```python
from build123d import *

# Parameters (mm, degrees)
SKETCH002_R  = 2.25
PAD002_DEPTH = 2
SKETCH003_W  = 7
SKETCH003_H  = 2
PAD003_DEPTH = 2
SKETCH004_W  = 32
SKETCH004_H  = 12
POCKET_DEPTH = 2


with BuildPart() as part:
    # Sketch002 → Pad002 (new body)
    with BuildSketch(Plane.XY):
        with BuildLine():
            Line((22.5, 12.5), (22.5, -12.5))
            Line((22.5, -12.5), (-5.5, -12.5))
            Line((-5.5, -12.5), (-5.5, -16.5))
            ThreePointArc((-15.5, -16.5), (-10.5, -21.5), (-5.5, -16.5))
            Line((-15.5, -12.5), (-15.5, -16.5))
            Line((-22.5, -12.5), (-15.5, -12.5))
            Line((-22.5, 12.5), (-22.5, -12.5))
            Line((-15.5, 12.5), (-22.5, 12.5))
            Line((-15.5, 16.5), (-15.5, 12.5))
            ThreePointArc((-5.5, 16.5), (-10.5, 21.5), (-15.5, 16.5))
            Line((-5.5, 16.5), (-5.5, 12.5))
            Line((-5.5, 12.5), (22.5, 12.5))
        make_face()
        with Locations((-10.5, 16.5)):
            Circle(SKETCH002_R, mode=Mode.SUBTRACT)
        with Locations((-10.5, -16.5)):
            Circle(SKETCH002_R, mode=Mode.SUBTRACT)
    extrude(amount=PAD002_DEPTH)

    # Sketch003 (on Face16 of Pad002) → Pad003 (join)
    with BuildSketch(Plane.XY.offset(2)):
        with Locations((19, -11.5)):
            Rectangle(SKETCH003_W, SKETCH003_H)
        Polygon((20.5, 10.5), (15.5, 10.5), (15.5, 12.5), (22.5, 12.5), (22.5, -0.5), (20.5, -0.5), align=None)
        Polygon((-15.5, 12.5), (-22.5, 12.5), (-22.5, -12.5), (-15.5, -12.5), (-15.5, -10.5), (-20.5, -10.5), (-20.5, 10.5), (-15.5, 10.5), align=None)
    extrude(amount=PAD003_DEPTH)

    # Sketch004 (on Face4 of Pad003) → Pocket (cut)
    with BuildSketch(Plane.XY.offset(2)):
        Rectangle(SKETCH004_W, SKETCH004_H)
    extrude(amount=-POCKET_DEPTH, mode=Mode.SUBTRACT)


solid = part.part
```
Verification items for the finished model (mm, model axes). A direction names the side the tool comes from. Coordinates: 2 decimals unless noted, no trailing zeros. Loops run counter-clockwise (first coordinate to the right, second up) from the corner with the lowest first, then second, coordinate; pieces in that order, holes last. Notation, with made-up numbers: (20, -36.75) -> (65, -36.75) arc R22 cw to (65, -20.75) -> close; hole circle Ø6 at (81.25, -39). An arc over 180 degrees is marked (long way). Put each result on its own line as item: value.
1. Gauge pin test, flat ends, axial feed: P1, Ø2, axis at y = 14, z = 1, coming from the -X side; P2, Ø4, axis at x = 15, y = -7, coming from the +Z side; P3, Ø2, axis at x = -20.5, z = 1, coming from the -Y side. Record the tip position at first contact, or that the pin passes through.
Result set:
P1: stops at x = -15.5
P2: stops at z = 2
P3: stops at y = -12.5
2. Thickness scan on line 1 (Y direction, x = -10.5, z = 0.7); line 2 (X direction, y = -3.5, z = 1); line 3 (Y direction, x = -1.5, z = 1.5). Record the ranges inside material, lowest first.
Result set:
line 1: y = -21.5 to -18.75, -14.25 to -6, 6 to 14.25, 18.75 to 21.5
line 2: x = -22.5 to -16, 16 to 22.5
line 3: y = -12.5 to -6, 6 to 12.5
3. Section check A-A, the plane y = -3.5. Record the boundary of the cut face in (x, z), then the cut area to 3 significant figures.
Result set:
outline: (-22.5, 0) -> (-16, 0) -> (-16, 2) -> (-20.5, 2) -> (-20.5, 4) -> (-22.5, 4) -> close; (16, 0) -> (22.5, 0) -> (22.5, 2) -> (16, 2) -> close
area: 30.0 mm^2
4. Section check D-D, the plane x = -10.5. Record the boundary of the cut face in (y, z).
Result set:
outline: (-21.5, 0) -> (-18.75, 0) -> (-18.75, 2) -> (-21.5, 2) -> close; (-14.25, 0) -> (-6, 0) -> (-6, 2) -> (-14.25, 2) -> close; (6, 0) -> (14.25, 0) -> (14.25, 2) -> (6, 2) -> close; (18.75, 0) -> (21.5, 0) -> (21.5, 2) -> (18.75, 2) -> close
5. Section check B-B, the plane x = 8. Record the boundary of the cut face in (y, z), then the cut area to 3 significant figures.
Result set:
outline: (-12.5, 0) -> (-6, 0) -> (-6, 2) -> (-12.5, 2) -> close; (6, 0) -> (12.5, 0) -> (12.5, 2) -> (6, 2) -> close
area: 26.0 mm^2
6. Mould release check, pull along X, two halves, no side actions. Record for faces 1 (the face through (-5.5, 15, 1)), 2 (the face through (0, -6, 1)), 3 (the face through (-10.4, 21.5, 1)): pulls with the +X half, pulls with the -X half, needs draft (parallel to the pull), parting line crosses it, or undercut.
Result set:
face 1: pulls with the +X half
face 2: undercut
face 3: parting line crosses it
7. Section check C-C, the plane z = 2.9. Record the boundary of the cut face in (x, y), then the cut area to 3 significant figures.
Result set:
outline: (-22.5, -12.5) -> (-15.5, -12.5) -> (-15.5, -10.5) -> (-20.5, -10.5) -> (-20.5, 10.5) -> (-15.5, 10.5) -> (-15.5, 12.5) -> (-22.5, 12.5) -> close; (15.5, -12.5) -> (22.5, -12.5) -> (22.5, -10.5) -> (15.5, -10.5) -> close; (15.5, 10.5) -> (20.5, 10.5) -> (20.5, -0.5) -> (22.5, -0.5) -> (22.5, 12.5) -> (15.5, 12.5) -> close
area: 120 mm^2
8. Tool access check on faces 4 (the face through (19, -10.5, 3)), 5 (the face through (-18, 10.5, 3)), 6 (the face through (11.4, -12.5, 1.5)), 7 (the face through (-15.5, -14, 1)), 8 (the face through (-15.5, -12, 3)). Record the directions out of +Z, -Z, +X, -X, +Y, -Y that give a thin tool (end or side, any length) a straight path to the whole face; none if there is none.
Result set:
face 4: +Z, +X
face 5: +Z
face 6: +Z, -Z, +X, -Y
face 7: +Z, -Z, -X, -Y
face 8: +Z, +Y, -Y
